Design review of the part built by this model. Coordinates are the model's own, in mm. A direction names the side the tool comes from. Give positions to 0.01 mm unless a question says otherwise; leave off trailing zeros. Write each loop counter-clockwise with the first axis right and the second up, starting at its lowest first coordinate (ties: lowest second). Pieces come first, ordered by that corner, then holes. Notation, with made-up numbers: (-24, 45) -> (-4, 45) arc R31 ccw to (-4, 81) -> close; hole circle Ø1 at (-35, 30.25). An arc over 180 degrees is marked (long way). Return JSON: item names as keys, results as strings. Group by question number.
from build123d import *

# Parameters (mm, degrees)
F0_R     = 31.75
F1_DEPTH = 25.4


with BuildPart() as f1:
    # F0 (on Top) → F1 (new body)
    with BuildSketch(Plane.XY):
        with BuildLine():
            Line((50.8, 6.35), (101.401368, 6.35))
            ThreePointArc((101.401368, 6.35), (98.137932, 26.296508), (90.990707, 45.202336))
            Line((90.990707, 45.202336), (47.267053, 19.958473))
            ThreePointArc((47.267053, 19.958473), (38.552563, 22.127038), (40.721129, 30.841527))
            ThreePointArc((40.721129, 30.841527), (40.819091, 30.899261), (40.918071, 30.955232))
            Line((40.918071, 30.955232), (84.641725, 56.199096))
            ThreePointArc((84.641725, 56.199096), (50.800442, 87.987926), (6.35, 101.401368))
            Line((6.35, 101.401368), (6.35, 50.8))
            ThreePointArc((6.35, 50.8), (0, 44.45), (-6.35, 50.8))
            Line((-6.35, 50.8), (-6.35, 101.401368))
            ThreePointArc((-6.35, 101.401368), (-50.800442, 87.987926), (-84.641725, 56.199096))
            Line((-84.641725, 56.199096), (-40.918071, 30.955232))
            ThreePointArc((-40.918071, 30.955232), (-38.523477, 28.62411), (-37.644091, 25.4))
            ThreePointArc((-37.644091, 25.4), (-40.76998, 19.929386), (-47.07011, 19.844768))
            ThreePointArc((-47.07011, 19.844768), (-47.169091, 19.900739), (-47.267053, 19.958473))
            Line((-47.267053, 19.958473), (-90.990707, 45.202336))
            ThreePointArc((-90.990707, 45.202336), (-98.137932, 26.296508), (-101.401368, 6.35))
            Line((-101.401368, 6.35), (-50.8, 6.35))
            ThreePointArc((-50.8, 6.35), (-46.309872, 4.490128), (-44.45, 0))
            ThreePointArc((-44.45, 0), (-46.309872, -4.490128), (-50.8, -6.35))
            Line((-50.8, -6.35), (-101.401368, -6.35))
            ThreePointArc((-101.401368, -6.35), (-71.842049, -71.842049), (-6.35, -101.401368))
            Line((-6.35, -101.401368), (-6.35, -50.8))
            ThreePointArc((-6.35, -50.8), (0, -44.45), (6.35, -50.8))
            Line((6.35, -50.8), (6.35, -101.401368))
            ThreePointArc((6.35, -101.401368), (71.842049, -71.842049), (101.401368, -6.35))
            Line((101.401368, -6.35), (50.8, -6.35))
            ThreePointArc((50.8, -6.35), (44.45, 0), (50.8, 6.35))
        make_face()
        Circle(F0_R, mode=Mode.SUBTRACT)
    extrude(amount=F1_DEPTH)


solid = f1.part
Q1. Take a section at C-C, the plane y = 39. Give the boundary of the cut face in (x, z), plus the area to 3 significant figures.
Q2. Insertion check: pin 1 (3 mm diameter, centred on y = -3.5, z = 2.5, fed in from +X); pin 2 (10 mm diameter, centred on x = -54, z = 19.5, fed in from +Y); pin 3 (12.5 mm diameter, centred on x = 66.5, z = 9, fed in from -Y). Each pin has a flat end and moves straight along its axis. Give the tip position at first contact, or say it passes through.
Q3. Take a section at A-A, the plane z = 18.75. Give the boundary of the cut face in (x, y).
Q4. Take a section at B-B, the plane y = 10. Give the boundary of the cut face in (x, z).
Q5. Tool access review of faces 1 (the face through (-6.35, -76, 13)), 2 (the face through (-76, 6.35, 13)), 3 (the face through (-6.35, 76, 13)): name each direction out of +Z, -Z, +X, -X, +Y, -Y from which nothing blocks a thin tool from reaching the whole face with its end or side.
Q6. Mouldability with a two-part tool opening along X and no side actions: class faces 4 (the face through (-24, -21.1, 25.4)), 5 (the face through (-72.565, -71.111, 12.522)), 6 (the face through (0.14, 44.45, 12.52)) as +X half, -X half, draft (parallel to the pull), parting line (faces both ways), or undercut.
Q7. For L1, parallel to Y at x = 0, z = 9.75; L2, parallel to X at y = 20, z = 5.5; L3, parallel to Y at x = -81.5, z = 24, list the stretches that pass through material, from the lowest coordinate up. Write a range as from..to.
Q8. Take a section at D-D, the plane y = 66.5. Give the boundary of the cut face in (x, z).
Final values:
{
 "1": {"outline": "(-93.82, 0) -> (-80.25, 0) -> (-80.25, 25.4) -> (-93.82, 25.4) -> close; (-54.85, 0) -> (54.85, 0) -> (54.85, 25.4) -> (-54.85, 25.4) -> close; (80.25, 0) -> (93.82, 0) -> (93.82, 25.4) -> (80.25, 25.4) -> close", "area": "3,480 mm²"},
 "2": {"pin 1": "stops at x = 46.89", "pin 2": "stops at y = 89", "pin 3": "stops at y = -81.81"},
 "3": {"outline": "(-101.4, -6.35) arc R101.6 ccw to (-6.35, -101.4) -> (-6.35, -50.8) arc R6.35 cw to (6.35, -50.8) -> (6.35, -101.4) arc R101.6 ccw to (101.4, -6.35) -> (50.8, -6.35) arc R6.35 cw to (50.8, 6.35) -> (101.4, 6.35) arc R101.6 ccw to (90.99, 45.2) -> (47.27, 19.96) arc R6.35 cw to (40.72, 30.84) arc R6.35 cw to (40.92, 30.96) -> (84.64, 56.2) arc R101.6 ccw to (6.35, 101.4) -> (6.35, 50.8) arc R6.35 cw to (-6.35, 50.8) -> (-6.35, 101.4) arc R101.6 ccw to (-84.64, 56.2) -> (-40.92, 30.96) arc R6.35 cw to (-37.64, 25.4) arc R6.35 cw to (-47.07, 19.84) arc R6.35 cw to (-47.27, 19.96) -> (-90.99, 45.2) arc R101.6 ccw to (-101.4, 6.35) -> (-50.8, 6.35) arc R6.35 cw to (-50.8, -6.35) -> close; hole circle Ø63.5 at (0, 0)"},
 "4": {"outline": "(-101.11, 0) -> (-30.13, 0) -> (-30.13, 25.4) -> (-101.11, 25.4) -> close; (30.13, 0) -> (101.11, 0) -> (101.11, 25.4) -> (30.13, 25.4) -> close"},
 "5": {"face 1": "+Z, -Z, -Y", "face 2": "+Z, -Z, -X", "face 3": "+Z, -Z, +Y"},
 "6": {"face 4": "draft", "face 5": "-X half", "face 6": "undercut"},
 "7": {"L1": "y = -44.45..-31.75, 31.75..44.45", "L2": "x = -99.61..-47.34, -40.65..-24.66, 24.66..40.65, 47.34..99.61", "L3": "y = -60.67..-6.35, 6.35..39.72, 54.39..60.67"},
 "8": {"outline": "(-76.81, 0) -> (-6.35, 0) -> (-6.35, 25.4) -> (-76.81, 25.4) -> close; (6.35, 0) -> (76.81, 0) -> (76.81, 25.4) -> (6.35, 25.4) -> close"}
}
